```python
from build123d import *

# Parameters (mm, degrees)
SKETCH2_R           = 1.5
SKETCH2_R_2         = 33
BOSS_EXTRUDE1_DEPTH = 2


with BuildPart() as part:
    # Sketch2 → Boss-Extrude1 (new body)
    with BuildSketch(Plane(origin=(0, 0, 0), x_dir=(1, 0, 0), z_dir=(0, 1, 0))):
        with BuildLine():
            Line((17.897079586, 48.929734976), (40.149284407, 43.651218265))
            ThreePointArc((40.149284407, 43.651218265), (42.540265174, 42.312242187), (43.866371506, 39.91409958))
            Line((43.866371506, 39.91409958), (49.02521675, 17.633846579))
            ThreePointArc((49.02521675, 17.633846579), (49.23478351, 16.809026698), (49.479249782, 15.993868858))
            ThreePointArc((49.479249782, 15.993868858), (51.999812242, -0.139738387), (49.392575566, -16.259565766))
            ThreePointArc((49.392575566, -16.259565766), (49.143731732, -17.073397941), (48.929734976, -17.897079586))
            Line((48.929734976, -17.897079586), (43.651218265, -40.149284407))
            ThreePointArc((43.651218265, -40.149284407), (42.312242187, -42.540265174), (39.91409958, -43.866371506))
            Line((39.91409958, -43.866371506), (17.633846579, -49.02521675))
            ThreePointArc((17.633846579, -49.02521675), (16.809026698, -49.23478351), (15.993868858, -49.479249782))
            ThreePointArc((15.993868858, -49.479249782), (-0.139738387, -51.999812242), (-16.259565766, -49.392575566))
            ThreePointArc((-16.259565766, -49.392575566), (-17.073397941, -49.143731732), (-17.897079586, -48.929734976))
            Line((-17.897079586, -48.929734976), (-40.149284407, -43.651218265))
            ThreePointArc((-40.149284407, -43.651218265), (-42.540265174, -42.312242187), (-43.866371506, -39.91409958))
            Line((-43.866371506, -39.91409958), (-49.02521675, -17.633846579))
            ThreePointArc((-49.02521675, -17.633846579), (-49.23478351, -16.809026698), (-49.479249782, -15.993868858))
            ThreePointArc((-49.479249782, -15.993868858), (-51.999812242, 0.139738387), (-49.392575566, 16.259565766))
            ThreePointArc((-49.392575566, 16.259565766), (-49.143731732, 17.073397941), (-48.929734976, 17.897079586))
            Line((-48.929734976, 17.897079586), (-43.651218265, 40.149284407))
            ThreePointArc((-43.651218265, 40.149284407), (-42.312242187, 42.540265174), (-39.91409958, 43.866371506))
            Line((-39.91409958, 43.866371506), (-17.633846579, 49.02521675))
            ThreePointArc((-17.633846579, 49.02521675), (-16.809026698, 49.23478351), (-15.993868858, 49.479249782))
            ThreePointArc((-15.993868858, 49.479249782), (-8.026622704, 51.3767781), (0.139738387, 51.999812242))
            ThreePointArc((0.139738387, 51.999812242), (8.302633013, 51.332896714), (16.259565766, 49.392575566))
            ThreePointArc((16.259565766, 49.392575566), (17.073397941, 49.143731732), (17.897079586, 48.929734976))
        make_face()
        with Locations(Location((-38.8907, 38.8907, 0), (0, 0, 270))):
            Circle(SKETCH2_R, mode=Mode.SUBTRACT)
        with Locations(Location((38.8907, 38.8907, 0), (0, 0, 90))):
            Circle(SKETCH2_R, mode=Mode.SUBTRACT)
        with Locations(Location((38.8907, -38.8907, 0), (0, 0, 270))):
            Circle(SKETCH2_R, mode=Mode.SUBTRACT)
        with Locations(Location((-38.8907, -38.8907, 0), (0, 0, 90))):
            Circle(SKETCH2_R, mode=Mode.SUBTRACT)
        with Locations(Location((0, 0, 0), (0, 0, 270))):
            Circle(SKETCH2_R_2, mode=Mode.SUBTRACT)
        with Locations(Location((0, 38.8907, 0), (0, 0, 270))):
            Circle(SKETCH2_R, mode=Mode.SUBTRACT)
        with Locations(Location((38.8907, 0, 0), (0, 0, 270))):
            Circle(SKETCH2_R, mode=Mode.SUBTRACT)
        with Locations(Location((0, -38.8907, 0), (0, 0, 270))):
            Circle(SKETCH2_R, mode=Mode.SUBTRACT)
        with Locations(Location((-38.8907, 0, 0), (0, 0, 270))):
            Circle(SKETCH2_R, mode=Mode.SUBTRACT)
    extrude(amount=BOSS_EXTRUDE1_DEPTH)


solid = part.part
```
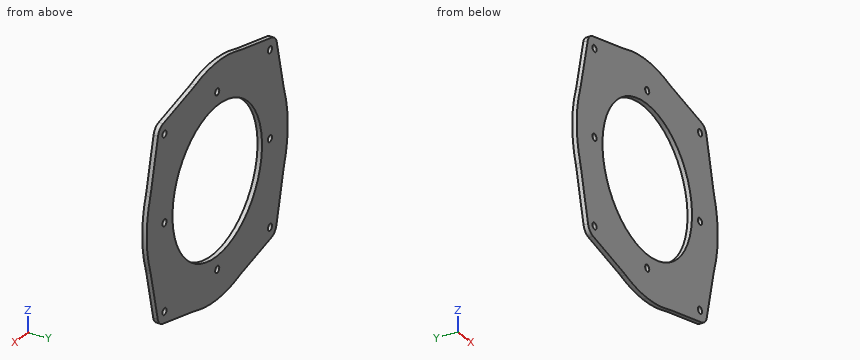
Source: CAD feature listing. Evaluate the final solid. Frame: model axes, mm. Round coordinates to 2 decimals unless told otherwise and drop trailing zeros. Loops run counter-clockwise (first coordinate to the right, second up) from the corner with the lowest first, then second, coordinate; pieces in that order, holes last. Notation, with made-up numbers: M -9,-5.5 L 23,-5.5 A16 ccw 23,18.5 Z; hole C 58.5,31.25 d1. An arc over 180 degrees is marked long. Use a Markdown table: item, result. Add a question column.
1. Cut plane B-B, the plane x = -8. Output: boundary loops of the cut face in (y, z).
2. Contact query for a flat-ended pin moving along its axis: pin 1 (2.5 mm diameter, centred on x = 0, z = -38.89, fed in from +Y). Output: stop coordinate, or through.
3. Cut plane C-C, the plane z = 13. Output: boundary loops of the cut face in (x, y).
4. Ray query, line 1 along X through (y, z) = (1.25, 0); line 2 along X through (y, z) = (0.3, 22); line 3 along Z through (x, y) = (6, 0.3). Return the intervals inside material, ascending. Write a range as [from, to].
5. Cut plane D-D, the plane y = 1. State how many separate pieces and enclosed holes the cut face has, and give its area (3 significant figures).
6. Cut plane A-A, the plane z = 0. Output: boundary loops of the cut face in (x, y).
Solution:
| question | item | result |
|---|---|---|
| 1 | outline | M 0,-51.38 L 2,-51.38 L 2,-32.02 L 0,-32.02 Z; M 0,32.02 L 2,32.02 L 2,51.38 L 0,51.38 Z |
| 2 | pin 1 | passes through |
| 3 | outline | M -50.35,0 L -30.33,0 L -30.33,2 L -50.35,2 Z; M 30.33,0 L 50.35,0 L 50.35,2 L 30.33,2 Z |
| 4 | line 1 | x = [-52, -40.39], [-37.39, -33], [33, 37.39], [40.39, 52] |
| 4 | line 2 | x = [-48.01, -24.6], [24.6, 47.96] |
| 4 | line 3 | z = [-51.65, -32.45], [32.45, 51.65] |
| 5 | separate pieces | 1 |
| 5 | enclosed holes | 9 |
| 5 | area | 5,650 mm2 |
| 6 | outline | M -52,0 L -40.39,0 L -40.39,2 L -52,2 Z; M -37.39,0 L -33,0 L -33,2 L -37.39,2 Z; M 33,0 L 37.39,0 L 37.39,2 L 33,2 Z; M 40.39,0 L 52,0 L 52,2 L 40.39,2 Z |
